```python
from build123d import *

# Parameters (mm, degrees)
BOSS_EXTRUDE1_DEPTH = 4.7625
SKETCH3_W           = 66.200858932
SKETCH3_H           = 5.079818348
BOSS_EXTRUDE2_DEPTH = 31.75
SKETCH4_W           = 28.999942
SKETCH4_H           = 12.9999994
CUT_EXTRUDE1_DEPTH  = 4.7625
SKETCH5_R           = 6.4999997
CUT_EXTRUDE2_DEPTH  = 4.7625
SKETCH6_R           = 3.175
CUT_EXTRUDE3_DEPTH  = 7.3025
SKETCH7_R           = 4.445
BOSS_EXTRUDE3_DEPTH = 14.605
SKETCH8_R           = 1.27
CUT_EXTRUDE4_DEPTH  = 50.8


with BuildPart() as part:
    # Sketch1 → Boss-Extrude1 (new body)
    with BuildSketch(Plane.XY):
        Polygon((30.222809818, 36.11360466), (25.142809818, 48.349181892), (-47.247190182, 48.349181892), (-52.327190182, 36.11360466), (-52.327190182, -53.715240876), (-47.247190182, -65.950818108), (25.142809818, -65.950818108), (30.222809818, -53.715240876), align=None)
    extrude(amount=BOSS_EXTRUDE1_DEPTH)

    # Sketch3 → Boss-Extrude2 (add)
    with BuildSketch(Plane.XY.offset(4.7625)):
        with Locations((-11.098760716, 45.809272718)):
            Rectangle(SKETCH3_W, SKETCH3_H)
        with Locations((-11.098760716, -63.410908934)):
            Rectangle(SKETCH3_W, SKETCH3_H)
    extrude(amount=BOSS_EXTRUDE2_DEPTH)

    # Sketch4 → Cut-Extrude1 (cut)
    with BuildSketch(Plane(origin=(0, 0, 0), x_dir=(-1, 0, 0), z_dir=(0, 0, -1))):
        with Locations((11.052190182, -27.850818108)):
            Rectangle(SKETCH4_W, SKETCH4_H)
    extrude(amount=-CUT_EXTRUDE1_DEPTH, mode=Mode.SUBTRACT)

    # Sketch5 → Cut-Extrude2 (cut)
    with BuildSketch(Plane(origin=(0, 0, 0), x_dir=(-1, 0, 0), z_dir=(0, 0, -1))):
        with Locations((11.052190182, 10.249181892)):
            Circle(SKETCH5_R)
    extrude(amount=-CUT_EXTRUDE2_DEPTH, mode=Mode.SUBTRACT)

    # Sketch6 → Cut-Extrude3 (cut)
    with BuildSketch(Plane.XZ.offset(65.950818108)):
        with Locations((-11.052190182, 20.6375)):
            Circle(SKETCH6_R)
    extrude(amount=-CUT_EXTRUDE3_DEPTH, mode=Mode.SUBTRACT)

    # Sketch7 → Boss-Extrude3 (add)
    with BuildSketch(Plane.XY.offset(4.7625)):
        with Locations((11.172809818, -40.550818108)):
            Circle(SKETCH7_R)
        with Locations((-33.277190182, -40.550818108)):
            Circle(SKETCH7_R)
        with Locations((11.172809818, 22.949181892)):
            Circle(SKETCH7_R)
        with Locations((-33.277190182, 22.949181892)):
            Circle(SKETCH7_R)
    extrude(amount=BOSS_EXTRUDE3_DEPTH)

    # Sketch8 → Cut-Extrude4 (cut)
    with BuildSketch(Plane.XY.offset(19.3675)):
        with Locations((-33.277190182, 22.949181892)):
            Circle(SKETCH8_R)
        with Locations((11.172809818, 22.949181892)):
            Circle(SKETCH8_R)
        with Locations((11.172809818, -40.550818108)):
            Circle(SKETCH8_R)
        with Locations((-33.277190182, -40.550818108)):
            Circle(SKETCH8_R)
    extrude(amount=-CUT_EXTRUDE4_DEPTH, mode=Mode.SUBTRACT)


solid = part.part
```
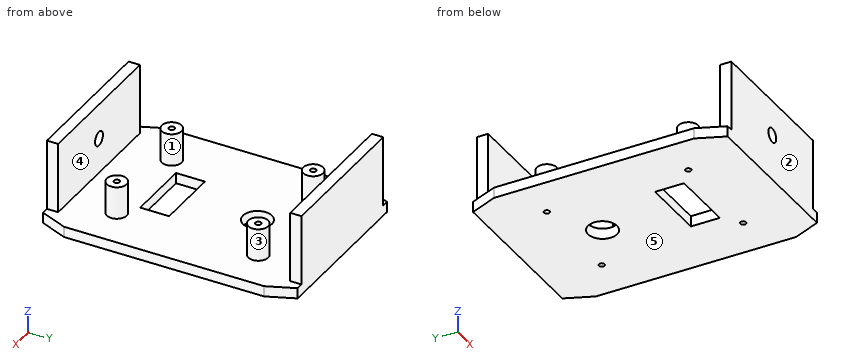
Here's how the part is built. I have some questions about the finished solid (model axes, mm). Face numbers are marked on the shaded views. A direction names the side the tool comes from. Give positions to 0.01 mm unless a question says otherwise; leave off trailing zeros. Write each loop counter-clockwise with the first axis right and the second up, starting at its lowest first coordinate (ties: lowest second). Pieces come first, ordered by that corner, then holes.
(1) Imagine slicing it at B-B, the plane x = 2. Write out the boundary of the cut face in (y, z).
Output values:
outline: (-65.95, 0) - (-34.35, 0) - (-34.35, 4.76) - (-60.87, 4.76) - (-60.87, 36.51) - (-65.95, 36.51) - close; (-21.35, 0) - (48.35, 0) - (48.35, 36.51) - (43.27, 36.51) - (43.27, 4.76) - (-21.35, 4.76) - close
(2) Imagine slicing it at A-A, the plane z = 25.5. Write out the boundary of the cut face in (x, y).
Output values:
outline: (-44.2, -65.95) - (22, -65.95) - (22, -60.87) - (-44.2, -60.87) - close; (-44.2, 43.27) - (22, 43.27) - (22, 48.35) - (-44.2, 48.35) - close
(3) If I drill on L1, parallel to Y at x = -16, z = 12.5; L2, parallel to Z at x = 3.5, y = -41.5; L3, parallel to Z at x = -35, y = 19, over which ranges is the centre line in solid material (lowest first)?
Output values:
L1: y = -65.95 to -60.87, 43.27 to 48.35
L2: z = 0 to 4.76
L3: z = 0 to 19.37
(4) Imagine slicing it at C-C, the plane y = -31. Write out the boundary of the cut face in (x, z), and give its area (3 significant figures).
Output values:
outline: (-52.33, 0) - (-25.55, 0) - (-25.55, 4.76) - (-52.33, 4.76) - close; (3.45, 0) - (30.22, 0) - (30.22, 4.76) - (3.45, 4.76) - close
area: 255 mm2
(5) On a 3-axis mill with a long thin cutter (end or side, diameter ignored), from which of +Z, -Z, +X, -X, +Y, -Y can I reach the whole of each face in a straight line? I mean the marked faces 3, 4 and 5. Say none if no direction works.
Output values:
face 3: +Z
face 4: +Z, +X, -X
face 5: -Z, +X, -X, +Y, -Y
(6) Imagine slicing it at D-D, the plane z = 14. Count the separate pieces of the cut face and the enclosed holes in it, and give its area (3 significant figures).
Output values:
separate pieces: 6
enclosed holes: 4
area: 901 mm2
(7) Will these pins go through, and if not, where does the flat tip stop? pin 1 (25 mm diameter, centred on x = 3.5, y = 2, fed in from +Z); pin 2 (10 mm diameter, centred on x = -33.5, y = 24.5, fed in from +Z); pin 3 (1 mm diameter, centred on x = -20.5, y = -53, fed in from -Z); pin 4 (1.5 mm diameter, centred on y = 45.5, z = 17.5, fed in from +X).
Output values:
pin 1: stops at z = 4.76
pin 2: stops at z = 19.37
pin 3: stops at z = 0
pin 4: stops at x = 22
(8) Thinking about a two-plate mould opening in X: for the marked faces 1 and 2, which applies, pulls with the +X half, pulls with the -X half, needs draft (parallel to the pull), parting line crosses it, or undercut?
Output values:
face 1: undercut
face 2: needs draft
